from build123d import *

# Parameters (mm, degrees)
F0_R     = 124.968
F0_W     = 127
F0_H     = 101.6
F1_DEPTH = 177.8


with BuildPart() as f1:
    # F0 (on Right) → F1 (new body)
    with BuildSketch(Plane.YZ):
        Circle(F0_R)
        Rectangle(F0_W, F0_H, mode=Mode.SUBTRACT)
    extrude(amount=F1_DEPTH)


solid = f1.part
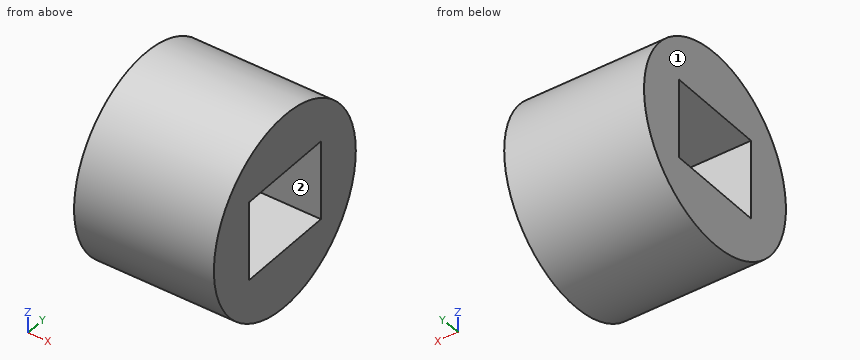
Verification items for the finished model (mm, model axes). Face numbers are marked on the shaded views. A direction names the side the tool comes from. Round coordinates to 2 decimals unless told otherwise and drop trailing zeros. Loops run counter-clockwise (first coordinate to the right, second up) from the corner with the lowest first, then second, coordinate; pieces in that order, holes last. Notation, with made-up numbers: (18.5, 86.25) - (31.5, 86.25) arc R31 ccw to (31.5, 117.25) - close; hole circle Ø5 at (3, 8.25). An arc over 180 degrees is marked (long way). Answer in a Markdown table with one row per item. Add a question column.
Q1. Tool access check on the marked faces 1 and 2. Record the directions out of +Z, -Z, +X, -X, +Y, -Y that give a thin tool (end or side, any length) a straight path to the whole face; none if there is none.
Q2. Section check D-D on y = 98.5. Enter the section's corners in (x, z), plus the area to 3 significant figures.
Q3. Section check A-A on z = 0. Enter the section's corners in (x, y), plus the area to 3 significant figures.
Q4. Gauge pin test, flat ends, axial feed: pin 1 (10 mm diameter, centred on x = 156, y = -71.5, fed in from +Z); pin 2 (8 mm diameter, centred on x = 54.5, y = 93, fed in from -Z); pin 3 (10 mm diameter, centred on x = 86.5, y = 40, fed in from -Z); pin 4 (10 mm diameter, centred on y = 22.5, z = 62, fed in from -X). Record the tip position at first contact, or that the pin passes through.
Q5. Section check C-C on x = 138. Enter the section's corners in (y, z), plus the area to 3 significant figures.
Q6. Material ranges on line 1 (Z direction, x = 85.5, y = -43.5); line 2 (Y direction, x = 98.5, z = -20); line 3 (Z direction, x = 85, y = -35.5), recorded low to high.
Q7. Section check B-B on y = 0. Enter the section's corners in (x, z), plus the area to 3 significant figures.
Found:
| question | item | result |
|---|---|---|
| 1 | face 1 | +Z, -Z, -X, +Y, -Y |
| 1 | face 2 | +X, -X |
| 2 | outline | (0, -76.91) - (177.8, -76.91) - (177.8, 76.91) - (0, 76.91) - close |
| 2 | area | 27,300 mm² |
| 3 | outline | (0, -124.97) - (177.8, -124.97) - (177.8, -63.5) - (0, -63.5) - close; (0, 63.5) - (177.8, 63.5) - (177.8, 124.97) - (0, 124.97) - close |
| 3 | area | 21,900 mm² |
| 4 | pin 1 | stops at z = 105.81 |
| 4 | pin 2 | stops at z = -87.73 |
| 4 | pin 3 | stops at z = -119.97 |
| 4 | pin 4 | stops at x = 0 |
| 5 | outline | circle Ø249.94 at (0, 0); hole (-63.5, -50.8) - (63.5, -50.8) - (63.5, 50.8) - (-63.5, 50.8) - close |
| 5 | area | 36,200 mm² |
| 6 | line 1 | z = -117.15 to -50.8, 50.8 to 117.15 |
| 6 | line 2 | y = -123.36 to -63.5, 63.5 to 123.36 |
| 6 | line 3 | z = -119.82 to -50.8, 50.8 to 119.82 |
| 7 | outline | (0, -124.97) - (177.8, -124.97) - (177.8, -50.8) - (0, -50.8) - close; (0, 50.8) - (177.8, 50.8) - (177.8, 124.97) - (0, 124.97) - close |
| 7 | area | 26,400 mm² |
